```python
from build123d import *

# Parameters (mm, degrees)
F0_R     = 5
F0_R_2   = 1.9
F1_DEPTH = 4.5
F2_DEPTH = 1
F3_SIZE  = 0.5


with BuildPart() as f1:
    # F0 (on Top) → F1 (new body)
    with BuildSketch(Plane.XY):
        Circle(F0_R)
        Circle(F0_R_2, mode=Mode.SUBTRACT)
    extrude(amount=F1_DEPTH)

    # F0 (on Top) → F2 (join)
    with BuildSketch(Plane.XY):
        Circle(F0_R_2)
    extrude(amount=F2_DEPTH)

    # F3
    f3_edges = [f1.edges().sort_by_distance(p)[0] for p in [
        (-5, 0, 4.5),
    ]]
    chamfer(f3_edges, length=F3_SIZE)


solid = f1.part
```
CAD build for the part. Positions are in the model's coordinates, mm. A direction names the side the tool comes from. Coordinates: 2 decimals unless noted, no trailing zeros. Loops run counter-clockwise (first coordinate to the right, second up) from the corner with the lowest first, then second, coordinate; pieces in that order, holes last. Notation, with made-up numbers: (77.25, 81.25) - (91.25, 81.25) arc R15 ccw to (91.25, 103.25) - close; hole circle Ø10 at (40.25, 85.5). An arc over 180 degrees is marked (long way). Use CSV: the item, a comma, the result in double quotes. Start each with the question number.
Q1. Two-plate mould, pull along X, no slides. Class faces 3 (the cylindrical face through (-1.08, -4.88, 1.97)), 4 (the cylindrical face through (-1.9, 0.08, 2.73)), 5 (the flat face through (1, -2, 4.5)): +X half, -X half, draft (parallel to the pull), parting line (faces both ways), or undercut.
Q2. Cut at A-A, the plane x = 0. List the corners of the cut face in (y, z), then the cut area to 4 significant figures.
Q3. Drop a flat-ended pin along its axis: P1, Ø2, axis at y = -3.5, z = 2, coming from the -X side. Give the stop position or say it passes through.
Q4. Cut at C-C, the plane z = 2. List the corners of the cut face in (x, y).
Q5. Cut at D-D, the plane z = 0.5. List the corners of the cut face in (x, y).
Q6. Probe probe 1 along Y at (x, z) = (0, 2.05); probe 2 along Y at (x, z) = (1, 2.55); probe 3 along X at (y, z) = (0.5, 2.4). List the from-to ranges inside material, lowest first. Write a range as from..to.
Q7. 3-axis set-ups, long thin cutter, end or side, ignore diameter. For faces 1 (the flat face through (0, 0, 0)), 2 (the flat face through (0, 0, 1)): which of +Z, -Z, +X, -X, +Y, -Y reach the whole face in a straight line?
Here are the results:
1,face 3,"parting line"
1,face 4,"undercut"
1,face 5,"draft"
2,outline,"(-5, 0) - (5, 0) - (5, 4) - (4.5, 4.5) - (1.9, 4.5) - (1.9, 1) - (-1.9, 1) - (-1.9, 4.5) - (-4.5, 4.5) - (-5, 4) - close"
2,area,"31.45 mm2"
3,P1,"x = -4.33"
4,outline,"circle Ø10 at (0, 0); hole circle Ø3.8 at (0, 0)"
5,outline,"circle Ø10 at (0, 0)"
6,probe 1,"-5..-1.9, 1.9..5"
6,probe 2,"-4.9..-1.62, 1.62..4.9"
6,probe 3,"-4.97..-1.83, 1.83..4.97"
7,face 1,"-Z, +X, -X, +Y, -Y"
7,face 2,"+Z"
